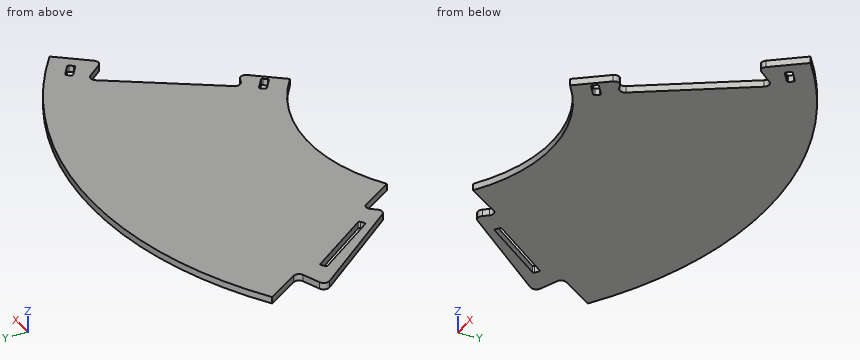
Autodesk Inventor part; units mm, degrees
ref_plane "YZ Plane" through (0, 0, 0) normal (1, 0, 0) x (0, 1, 0)
ref_plane "XZ Plane" through (0, 0, 0) normal (0, 1, 0) x (-1, 0, 0)
ref_plane "XY Plane" through (0, 0, 0) normal (0, 0, 1) x (1, 0, 0)
sketch "CONTOURS" plane through (0, 0, 0) normal (0, 0, 1) x (1, 0, 0)
  arc A0 (1467.8843, 188.4261) -> (1444.4964, 189.5904) centre (1455.765, 180.4653) ccw
  line L0 (1444.4964, 189.5904) -> (1433.8001, 176.3815)
  arc A1 (1409.6695, 176.43) -> (1433.8001, 176.3815) centre (1421.7543, 186.136) ccw
  line L1 (1409.6695, 176.43) -> (1205.1516, 431.0714)
  arc A2 (1211.6817, 455.248) -> (1205.1516, 431.0714) centre (1217.2364, 440.7775) ccw
  line L2 (1211.6817, 455.248) -> (1259.5115, 473.6081)
  arc A3 (1259.5115, 473.6081) -> (1266.4344, 495.1059) centre (1254.3152, 487.1451) ccw
  line L3 (1266.4344, 495.1059) -> (1206.4511, 586.4222)
  arc A4 (2416.4096, 529.2878) -> (1206.4511, 586.4222) centre (1772.0714, -275.6668) ccw
  line L4 (2416.4096, 529.2878) -> (2348.9296, 445.0595)
  arc A5 (2326.3448, 445.0004) -> (2348.9296, 445.0595) centre (2337.6134, 454.1255) ccw
  line L5 (2326.3448, 445.0004) -> (2294.0217, 484.916)
  arc A6 (2294.0217, 484.916) -> (2269.0106, 483.6555) centre (2281.976, 475.1615) ccw
  line L6 (2269.0106, 483.6555) -> (2088.6011, 208.2752)
  arc A7 (2088.6011, 208.2752) -> (2096.0118, 185.3107) centre (2101.5665, 199.7812) ccw
  line L7 (2096.0118, 185.3107) -> (2111.7592, 179.2658)
  arc A8 (2117.8791, 156.6628) -> (2111.7592, 179.2658) centre (2106.5629, 165.7289) ccw
  line L8 (2117.8791, 156.6628) -> (2053.1174, 75.8275)
  arc A9 (2053.1174, 75.8275) -> (1525.5022, 100.7107) centre (1772.1395, -275.8029) ccw
  line L9 (1525.5022, 100.7107) -> (1467.8843, 188.4261)
sketch "HOLES" plane through (0, 0, 0) normal (0, 0, 1) x (1, 0, 0)
  line L0 (2054.9481, 158.6603) -> (2084.0727, 137.5)
  arc A0 (2084.9576, 131.9128) -> (2084.0727, 137.5) centre (2081.7215, 134.264) ccw
  line L1 (2084.9576, 131.9128) -> (2078.492, 123.0136)
  arc A1 (2072.9048, 122.1287) -> (2078.492, 123.0136) centre (2075.2559, 125.3648) ccw
  line L2 (2072.9048, 122.1287) -> (2043.7801, 143.289)
  arc A2 (2042.8952, 148.8762) -> (2043.7801, 143.289) centre (2046.1313, 146.5251) ccw
  line L3 (2042.8952, 148.8762) -> (2049.3609, 157.7754)
  arc A3 (2054.9481, 158.6603) -> (2049.3609, 157.7754) centre (2052.5969, 155.4242) ccw
  line L4 (1405.0745, 238.9064) -> (1396.1753, 232.4408)
  arc A4 (1390.5881, 233.3257) -> (1396.1753, 232.4408) centre (1393.8242, 235.6768) ccw
  line L5 (1390.5881, 233.3257) -> (1267.741, 402.4102)
  arc A5 (1268.6259, 407.9975) -> (1267.741, 402.4102) centre (1270.9771, 404.7614) ccw
  line L6 (1268.6259, 407.9975) -> (1277.5251, 414.4631)
  arc A6 (1283.1123, 413.5782) -> (1277.5251, 414.4631) centre (1279.8762, 411.227) ccw
  line L7 (1283.1123, 413.5782) -> (1405.9594, 244.4936)
  arc A7 (1405.0745, 238.9064) -> (1405.9594, 244.4936) centre (1402.7234, 242.1425) ccw
  line L8 (2316.1678, 525.0037) -> (2322.6335, 533.9029)
  arc A8 (2328.2207, 534.7878) -> (2322.6335, 533.9029) centre (2325.8696, 531.5518) ccw
  line L9 (2328.2207, 534.7878) -> (2357.3453, 513.6276)
  arc A9 (2358.2302, 508.0403) -> (2357.3453, 513.6276) centre (2354.9942, 510.3915) ccw
  line L10 (2358.2302, 508.0403) -> (2351.7646, 499.1412)
  arc A10 (2346.1774, 498.2562) -> (2351.7646, 499.1412) centre (2348.5285, 501.4923) ccw
  line L11 (2346.1774, 498.2562) -> (2317.0528, 519.4165)
  arc A11 (2316.1678, 525.0037) -> (2317.0528, 519.4165) centre (2319.4039, 522.6526) ccw
sketch "LETTERS" plane through (0, 0, 0) normal (0, 0, 1) x (1, 0, 0)
  line L0 (2123.0862, 379.0631) -> (2113.6777, 384.09)
  line L1 (2105.5346, 377.443) -> (2118.4889, 370.5215)
  line L2 (2118.4889, 370.5215) -> (2127.8234, 387.992)
extrude "Extrusion3" add sketch "CONTOURS" along normal blind 18
extrude "Extrusion4" cut sketch "HOLES" along normal blind 18
properties part number "Platform F3" material "Wood (Birch)"
Geometry: final body of the model. Coordinates: model frame, mm. Round coordinates to 2 decimals unless told otherwise and drop trailing zeros. Write each loop counter-clockwise with the first axis right and the second up, starting at its lowest first coordinate (ties: lowest second). Pieces come first, ordered by that corner, then holes. Notation, with made-up numbers: M -0.75,-9.5 L 10.25,-9.5 A22 ccw 10.25,20.5 Z; hole C -11,82 d5. An arc over 180 degrees is marked long. Answer in a Markdown table with one row per item. Add a question column.
(1) Cut plane D-D, the plane x = 2224.5. Return the cut outline in (y, z), then the cut area to 3 significant figures.
(2) Cut plane B-B, the plane x = 1364. Return the cut outline in (y, z), then the cut area to 3 significant figures.
(3) Cut plane A-A, the plane y = 342. Return the cut outline in (x, z), then the cut area to 3 significant figures.
(4) Contact query for flat-ended pins moving along their axis: pin 1 (2 mm diameter, centred on y = 635.5, z = 8.5, fed in from -X); pin 2 (1 mm diameter, centred on x = 2225.5, z = 3.5, fed in from -Y); pin 3 (1 mm diameter, centred on x = 1534, z = 7, fed in from -Y). Output: stop coordinate, or through.
(5) Cut plane C-C, the plane z = 3.25. Give the number of separate pieces and of enclosed holes in the cut face, then the cut area to 3 significant figures.
(6) Ray query, L1, parallel to X at y = 524, z = 13.5; L2, parallel to Y at x = 2090, z = 12.75; L3, parallel to X at y = 355, z = 1. Return the intervals inside material, ascending.
Established:
| question | item | result |
|---|---|---|
| 1 | outline | M 415.71,0 L 650.85,0 L 650.85,18 L 415.71,18 Z |
| 1 | area | 4,230 mm² |
| 2 | outline | M 233.29,0 L 269.92,0 L 269.92,18 L 233.29,18 Z; M 302.25,0 L 671.22,0 L 671.22,18 L 302.25,18 Z |
| 2 | area | 7,300 mm² |
| 3 | outline | M 1276.69,0 L 1311.63,0 L 1311.63,18 L 1276.69,18 Z; M 1335.12,0 L 2176.21,0 L 2176.21,18 L 1335.12,18 Z |
| 3 | area | 15,800 mm² |
| 4 | pin 1 | x = 1287.59 |
| 4 | pin 2 | y = 416.48 |
| 4 | pin 3 | y = 105.83 |
| 5 | separate pieces | 1 |
| 5 | enclosed holes | 3 |
| 5 | area | 534,000 mm² |
| 6 | L1 | 1247.45 to 2315.64, 2343.07 to 2412.17 |
| 6 | L2 | 121.86 to 189.46, 210.41 to 705.17 |
| 6 | L3 | 1266.25 to 1302.19, 1325.67 to 2184.72 |
